```python
from build123d import *

# Parameters (mm, degrees)
BOSS_EXTRUDE1_DEPTH     = 10
SKETCH3_W               = 76
SKETCH3_H               = 5.65
SKETCH4_W               = 14
SKETCH4_H               = 14
BOSS_EXTRUDE2_DEPTH     = 10
SKETCH5_W               = 10
SKETCH5_H               = 10
CUT_EXTRUDE1_DEPTH      = 8
CUT_EXTRUDE1_DEPTH_BACK = 8
HOLE1_D                 = 4.134
HOLE1_DEPTH             = 7
HOLE1_CSINK_D           = 5
HOLE1_CSINK_ANGLE       = 90
HOLE2_D                 = 4.134
HOLE2_DEPTH             = 8
HOLE2_CSINK_D           = 5
HOLE2_CSINK_ANGLE       = 90
HOLE2_TIP               = 1.193383006


with BuildPart() as part:
    # Sketch1 → Revolve1 (revolve)
    with BuildSketch(Plane.XY):
        with BuildLine():
            Line((0, 0), (0, 5.15))
            Line((0, 5.15), (0.85, 6))
            Line((0.85, 6), (7.35, 6))
            Line((7.35, 6), (8.174264069, 5.175735931))
            ThreePointArc((8.174264069, 5.175735931), (8.368918078, 5.04567228), (8.598528137, 5))
            Line((8.598528137, 5), (9.4, 5))
            ThreePointArc((9.4, 5), (9.824264069, 5.175735931), (10, 5.6))
            Line((10, 5.6), (10, 6))
            Line((10, 6), (12, 6))
            Line((12, 6), (12, 0))
            Line((12, 0), (0, 0))
        make_face()
    revolve(axis=Axis((12, 0, 0), (-1, 0, 0)))

    # Sketch2 → Boss-Extrude1 (add)
    with BuildSketch(Plane(origin=(12, 0, 0), x_dir=(0, 0, -1), z_dir=(1, 0, 0))):
        with BuildLine():
            Line((-3.872983346, -7), (3.872983346, -7))
            ThreePointArc((3.872983346, -7), (5.656854249, -5.656854249), (7, -3.872983346))
            Line((7, -3.872983346), (7, 3.872983346))
            ThreePointArc((7, 3.872983346), (5.656854249, 5.656854249), (3.872983346, 7))
            Line((3.872983346, 7), (-3.872983346, 7))
            ThreePointArc((-3.872983346, 7), (-5.656854249, 5.656854249), (-7, 3.872983346))
            Line((-7, 3.872983346), (-7, -3.872983346))
            ThreePointArc((-7, -3.872983346), (-5.656854249, -5.656854249), (-3.872983346, -7))
        make_face()
    extrude(amount=BOSS_EXTRUDE1_DEPTH)

    # Sketch3 → Revolve2 (revolve)
    with BuildSketch(Plane.XY):
        with Locations((60, 2.825)):
            Rectangle(SKETCH3_W, SKETCH3_H)
    revolve(axis=Axis((98, 0, 0), (-1, 0, 0)))

    # Sketch4 → Boss-Extrude2 (add)
    with BuildSketch(Plane(origin=(98, 0, 0), x_dir=(0, 0, -1), z_dir=(1, 0, 0))):
        Rectangle(SKETCH4_W, SKETCH4_H)
    extrude(amount=BOSS_EXTRUDE2_DEPTH)

    # Sketch5 → Cut-Revolve1 (revolve, cut)
    with BuildSketch(Plane.XY):
        with Locations((103, 13)):
            Rectangle(SKETCH5_W, SKETCH5_H)
    revolve(axis=Axis((108, 0, 0), (-1, 0, 0)), mode=Mode.SUBTRACT)

    # Sketch6 → Revolve3 (revolve)
    with BuildSketch(Plane.XY):
        with BuildLine():
            Line((108, 0), (108, 6))
            Line((108, 6), (110, 6))
            Line((110, 6), (110, 5.6))
            ThreePointArc((110, 5.6), (110.175735931, 5.175735931), (110.6, 5))
            Line((110.6, 5), (111.401471863, 5))
            ThreePointArc((111.401471863, 5), (111.631081922, 5.04567228), (111.825735931, 5.175735931))
            Line((111.825735931, 5.175735931), (112.65, 6))
            Line((112.65, 6), (119.15, 6))
            Line((119.15, 6), (120, 5.15))
            Line((120, 5.15), (120, 0))
            Line((120, 0), (108, 0))
        make_face()
    revolve(axis=Axis((120, 0, 0), (-1, 0, 0)))

    # Sketch7 → Cut-Extrude1 (cut, two sides)
    with BuildSketch(Plane(origin=(0, 0, 0), x_dir=(1, 0, 0), z_dir=(0, 1, 0))) as cut_extrude1_sk:
        Polygon((104, 12), (104, 4), (120, 4), (120, -4), (104, -4), (104, -12), (128, -12), (128, 12), align=None)
    extrude(amount=CUT_EXTRUDE1_DEPTH, mode=Mode.SUBTRACT)
    extrude(cut_extrude1_sk.sketch, amount=-CUT_EXTRUDE1_DEPTH_BACK, mode=Mode.SUBTRACT)

    # Sketch8 → Cut-Revolve2 (revolve, cut)
    with BuildSketch(Plane(origin=(110, 0, 0), x_dir=(0, 0, -1), z_dir=(1, 0, 0))):
        Polygon((-4.2, 0), (-4.2, 3.192820323), (-3, 2.5), (-3.5, 2.5), (-4, 2.211324865), (-4, 2), (4, 2), (4, 2.211324865), (3.5, 2.5), (3, 2.5), (4.2, 3.192820323), (4.2, 0), align=None)
    revolve(axis=Axis((110, 0, -4), (0, 0, 1)), mode=Mode.SUBTRACT)

    # Hole1
    with Locations(Plane(origin=(0, 7, 0), x_dir=(1, 0, 0), z_dir=(0, 1, 0))):
        with Locations((18, 0)):
            CounterSinkHole(HOLE1_D / 2, HOLE1_CSINK_D / 2, depth=HOLE1_DEPTH, counter_sink_angle=HOLE1_CSINK_ANGLE)

    # Hole2
    with Locations(Plane(origin=(0, 7, 0), x_dir=(1, 0, 0), z_dir=(0, 1, 0))):
        with Locations((102, 0)):
            CounterSinkHole(HOLE2_D / 2, HOLE2_CSINK_D / 2, depth=HOLE2_DEPTH, counter_sink_angle=HOLE2_CSINK_ANGLE)
            with Locations((0, 0, -(HOLE2_DEPTH + HOLE2_TIP / 2))):  # 120° drill point
                Cone(0, HOLE2_D / 2, HOLE2_TIP, mode=Mode.SUBTRACT)

    # Sketch13 → Cut-Revolve3 (revolve, cut)
    with BuildSketch(Plane.XY):
        Polygon((-4, 0), (-4, 2), (31.5, 2), (31.5, 5), (84, 5), (84, 0), align=None)
    revolve(axis=Axis((84, 0, 0), (-1, 0, 0)), mode=Mode.SUBTRACT)


solid = part.part
```
Input: part model. Units: mm. Frame: model coordinates. A direction names the side the tool comes from. Give positions to 0.01 mm unless a question says otherwise; leave off trailing zeros. Write each loop counter-clockwise with the first axis right and the second up, starting at its lowest first coordinate (ties: lowest second). Pieces come first, ordered by that corner, then holes. Notation, with made-up numbers: (-1.75, 18.25) - (10.25, 18.25) arc R16 ccw to (10.25, 49.25) - close; hole circle Ø1 at (-13, 55). An arc over 180 degrees is marked (long way). Write item = value, one per line. Start each with the question number.
1) Draft query along X for faces 1 (the face through (4, -6, 0)), 2 (the face through (110, -5.8, 0)), 3 (the face through (119.86, 5.29, 0.07)). Return one class per face: pulls with the +X half, pulls with the -X half, needs draft (parallel to the pull), parting line crosses it, or undercut.
2) Cut plane A-A (x = 34.5). Return loops of the section in (y, z), and give its area (3 significant figures).
3) Pin query (flat end, axial travel): pin 1 (1 mm diameter, centred on x = 23, z = -3, fed in from -Y); pin 2 (2 mm diameter, centred on x = 51.5, y = -2, fed in from +Z); pin 3 (3 mm diameter, centred on x = 106.5, y = -2, fed in from +Z); pin 4 (1.3 mm diameter, centred on x = 109.5, y = 0, fed in from +Z). Return the tip coordinate at first contact, or that it passes through.
4) Material intervals for L1, parallel to X at y = 5.5, z = -3.5; L2, parallel to Y at x = 39.5, z = 0.25; L3, parallel to X at y = 4, z = -6, sorted ascending. Write a range as [from, to].
5) Reachability of faces 4 (the face through (16, -2, 0)), 5 (the face through (101, 0, -7)), 6 (the face through (10, 5, -3)), 7 (the face through (106, 0, -4)), 8 (the face through (116, 0, 4)) from +Z, -Z, +X, -X, +Y, -Y: full face, straight path, thin tool, end or side. Return the list, or none.
6) Cut plane B-B (x = 91.5). Return loops of the section in (y, z).
Answers follow:
q1.face_1 = needs draft
q1.face_2 = undercut
q1.face_3 = pulls with the +X half
q2.outline = circle Ø11.3 at (0, 0); hole circle Ø10 at (0, 0)
q2.area = 21.7 mm^2
q3.pin_1 = -5.07
q3.pin_2 = 5.56
q3.pin_3 = 4
q3.pin_4 = through
q4.L1 = [12, 22], [98, 108]
q4.L2 = [-5.64, -4.99], [4.99, 5.64]
q4.L3 = [12, 22], [98, 104]
q5.face_4 = -X
q5.face_5 = -Z, +X, -X, +Y, -Y
q5.face_6 = none
q5.face_7 = -Z, +X, +Y, -Y
q5.face_8 = +Z, +X, +Y, -Y
q6.outline = circle Ø11.3 at (0, 0)
